```python
from build123d import *

# Parameters (mm, degrees)
F1_DEPTH      = 2
F2_R          = 2
F2_R_2        = 1
F3_DEPTH      = 4.325
F3_DEPTH_BACK = 4.325
F4_W          = 0.9
F4_H          = 2.5
F5_DEPTH      = 3.00062


with BuildPart() as f1:
    # F0 (on Top) → F1 (new body)
    with BuildSketch(Plane.XY):
        Polygon((0, 18.958714), (17, 18.958714), (17, 24.958714), (10.25, 44.958714), (0, 44.958714), (-10.25, 44.958714), (-17, 24.958714), (-17, 18.958714), align=None)
    extrude(amount=F1_DEPTH)

    # F2 (on Right) → F3 (join, two sides)
    with BuildSketch(Plane.YZ) as f3_sk:
        with Locations((17.221542, 1.00038)):
            Circle(F2_R)
        with Locations((17.221542, 1.00038)):
            Circle(F2_R_2, mode=Mode.SUBTRACT)
    extrude(amount=F3_DEPTH)
    extrude(f3_sk.sketch, amount=-F3_DEPTH_BACK)

    # F4 (on face) → F5 (cut, through all)
    with BuildSketch(Plane.XY.offset(2)):
        with Locations((-4.775, 20.208714)):
            Rectangle(F4_W, F4_H)
        with Locations((4.775, 20.208714)):
            Rectangle(F4_W, F4_H)
    extrude(amount=-F5_DEPTH, mode=Mode.SUBTRACT)


solid = f1.part
```
The model under review builds one solid part; all positions refer to its coordinate system, in mm. A direction names the side the tool comes from. Round coordinates to 2 decimals unless told otherwise and drop trailing zeros. Order: outer loops, then holes, each group sorted by start corner. A loop starts at its lowest first (then second) coordinate and runs counter-clockwise, first axis right, second up.
Item 1: Machinability: for faces 1 (the flat face through (-5, 21.459, 1)), 2 (the flat face through (0, 32, 0)), 3 (the flat face through (0, 32, 2)), which of the approach directions +Z, -Z, +X, -X, +Y, -Y give a long, thin tool a straight path to every point of the face, cutting with its end or side? Answer none if there is none.
Working result:
face 1: +Z, -Z, -Y
face 2: -Z, +X, -X, +Y
face 3: +Z, +X, -X, +Y
Item 2: Draft analysis for pull direction X (two halves, no side actions). For faces 4 (the flat face through (5, 21.459, 1)), 5 (the flat face through (13.67, 34.82, 0.99)), 6 (the flat face through (0, 44.959, 1)), state which applies: released by +X, released by -X, zero draft, split by the parting line, or undercut.
Working result:
face 4: undercut
face 5: released by +X
face 6: zero draft
Item 3: Add section A-A, the plane y = 19.5. State the section outline as (x, z) points (3 decimals), and give its area (3 significant figures).
Working result:
outline: (-17, 0) - (-5.225, 0) - (-5.225, 2) - (-17, 2) - close; (-4.325, 0) - (4.325, 0) - (4.325, 2) - (-4.325, 2) - close; (5.225, 0) - (17, 0) - (17, 2) - (5.225, 2) - close
area: 64.4 mm2
Item 4: Add section B-B, the plane z = 0.6. State the section outline as (x, y) points (3 decimals), and give its area (3 significant figures).
Working result:
outline: (-17, 18.959) - (-5.225, 18.959) - (-5.225, 21.459) - (-4.325, 21.459) - (-4.325, 18.138) - (4.325, 18.138) - (4.325, 21.459) - (5.225, 21.459) - (5.225, 18.959) - (17, 18.959) - (17, 24.959) - (10.25, 44.959) - (-10.25, 44.959) - (-17, 24.959) - close; (-4.325, 15.262) - (4.325, 15.262) - (4.325, 16.305) - (-4.325, 16.305) - close
area: 761 mm2
Item 5: For pin 1 (13 mm diameter, centred on x = -7, y = 29.5, fed in from +Z); pin 2 (1 mm diameter, centred on x = 13.5, z = 1, fed in from -Y); pin 3 (1.2 mm diameter, centred on y = 17.5, z = 1.5, fed in from +X) (3 decimals); pin 4 (2 mm diameter, centred on y = 18, z = 0.5, fed in from -X), all flat-tipped, find the tip position at first contact; note any pin that passes through.
Working result:
pin 1: stops at z = 2
pin 2: stops at y = 18.96
pin 3: stops at x = 4.325
pin 4: stops at x = -17
Item 6: To check wall thickness, follow probe 1 along Z at (x, y) = (-11, 31.75); probe 2 along Y at (x, z) = (9, 0.05); probe 3 along Y at (x, z) = (4.5, 1.3). State the ranges of each line that lie inside material, in increasing order.
Working result:
probe 1: z = 0 to 2
probe 2: y = 18.96 to 44.96
probe 3: y = 21.46 to 44.96
Item 7: Add section D-D, the plane x = 7. State the section outline as (y, z) points.
Working result:
outline: (18.96, 0) - (44.96, 0) - (44.96, 2) - (18.96, 2) - close
